For this review, take the finished solid that the model builds, in its own axes (mm). Coordinates: 2 decimals unless noted, no trailing zeros. Loops run counter-clockwise (first coordinate to the right, second up) from the corner with the lowest first, then second, coordinate; pieces in that order, holes last. Notation, with made-up numbers: (18, 22) -> (55, 22) arc R22 cw to (55, 34) -> close; hole circle Ø9 at (27, 53). An arc over 180 degrees is marked (long way). Answer in a Markdown table with one row per item.
from build123d import *

# Parameters (mm, degrees)
SKETCH_1_W          = 53
SKETCH_1_H          = 40
EXTRUDE_1_DEPTH     = 3
SKETCH_2_R          = 1.55
CUT_EXTRUDE_1_DEPTH = 10
SKETCH_4_R          = 1.65
CUT_EXTRUDE_2_DEPTH = 10
SKETCH_5_R          = 1.05
CUT_EXTRUDE_3_DEPTH = 10
SKETCH_6_W          = 23
SKETCH_6_H          = 12.5
CUT_EXTRUDE_4_DEPTH = 10
SKETCH_7_W          = 24
SKETCH_7_H          = 14
CUT_EXTRUDE_5_DEPTH = 10
SKETCH_8_W          = 40
SKETCH_8_H          = 10
CUT_EXTRUDE_6_DEPTH = 10
SKETCH_9_R          = 1.55
CUT_EXTRUDE_7_DEPTH = 10
FILLET_1_R          = 2


with BuildPart() as part:
    # 草图1 → 凸台-拉伸1 (new body)
    with BuildSketch(Plane(origin=(0, 0, 0), x_dir=(1, 0, 0), z_dir=(0, 1, 0))):
        Rectangle(SKETCH_1_W, SKETCH_1_H)
    extrude(amount=EXTRUDE_1_DEPTH)

    # 草图2 → 切除-拉伸1 (cut)
    with BuildSketch(Plane(origin=(0, 0, 0), x_dir=(-1, 0, 0), z_dir=(0, -1, 0))):
        with Locations(Location((20.5, -15, 0), (0, 0, 90))):
            Circle(SKETCH_2_R)
        with Locations(Location((20.5, 5, 0), (0, 0, 90))):
            Circle(SKETCH_2_R)
    extrude(amount=-CUT_EXTRUDE_1_DEPTH, mode=Mode.SUBTRACT)

    # 草图4 → 切除-拉伸2 (cut)
    with BuildSketch(Plane(origin=(0, 3, 0), x_dir=(1, 0, 0), z_dir=(0, 1, 0))):
        with Locations(Location((-8.5, -17, 0), (0, 0, 270))):
            Circle(SKETCH_4_R)
        with Locations(Location((11.5, -17, 0), (0, 0, 270))):
            Circle(SKETCH_4_R)
        with Locations(Location((-0.5, 17, 0), (0, 0, 270))):
            Circle(SKETCH_4_R)
        with Locations(Location((19.5, 17, 0), (0, 0, 270))):
            Circle(SKETCH_4_R)
    extrude(amount=-CUT_EXTRUDE_2_DEPTH, mode=Mode.SUBTRACT)

    # 草图5 → 切除-拉伸3 (cut)
    with BuildSketch(Plane(origin=(0, 3, 0), x_dir=(1, 0, 0), z_dir=(0, 1, 0))):
        with Locations(Location((22.599975, -7.75, 0), (0, 0, 270))):
            Circle(SKETCH_5_R)
        with Locations(Location((-5.100025, -7.75, 0), (0, 0, 270))):
            Circle(SKETCH_5_R)
    extrude(amount=-CUT_EXTRUDE_3_DEPTH, mode=Mode.SUBTRACT)

    # 草图6 → 切除-拉伸4 (cut)
    with BuildSketch(Plane(origin=(0, 0, 0), x_dir=(-1, 0, 0), z_dir=(0, -1, 0))):
        with Locations((-8.749975, -7.75)):
            Rectangle(SKETCH_6_W, SKETCH_6_H)
    extrude(amount=-CUT_EXTRUDE_4_DEPTH, mode=Mode.SUBTRACT)

    # 草图7 → 切除-拉伸5 (cut)
    with BuildSketch(Plane(origin=(0, 0, 0), x_dir=(-1, 0, 0), z_dir=(0, -1, 0))):
        with Locations((-8.749975, -7.75)):
            Rectangle(SKETCH_7_W, SKETCH_7_H)
    extrude(amount=-CUT_EXTRUDE_5_DEPTH, mode=Mode.SUBTRACT)

    # 草图8 → 切除-拉伸6 (cut)
    with BuildSketch(Plane(origin=(0, 0, 0), x_dir=(-1, 0, 0), z_dir=(0, -1, 0))):
        with Locations((-6.5, 15)):
            Rectangle(SKETCH_8_W, SKETCH_8_H)
    extrude(amount=-CUT_EXTRUDE_6_DEPTH, mode=Mode.SUBTRACT)

    # 草图9 → 切除-拉伸7 (cut)
    with BuildSketch(Plane(origin=(0, 0, 0), x_dir=(-1, 0, 0), z_dir=(0, -1, 0))):
        with Locations(Location((-11.5, 7, 0), (0, 0, 90))):
            Circle(SKETCH_9_R)
        with Locations(Location((8.5, 7, 0), (0, 0, 90))):
            Circle(SKETCH_9_R)
    extrude(amount=-CUT_EXTRUDE_7_DEPTH, mode=Mode.SUBTRACT)

    # 圆角1
    fillet_1_edges = [part.edges().sort_by_distance(p)[0] for p in [
        (26.5, 1.5, -10),
        (-13.5, 1.5, -20),
        (-13.5, 1.5, -10),
        (26.5, 1.5, 20),
        (-26.5, 1.5, 20),
        (-26.5, 1.5, -20),
    ]]
    fillet(fillet_1_edges, radius=FILLET_1_R)


solid = part.part
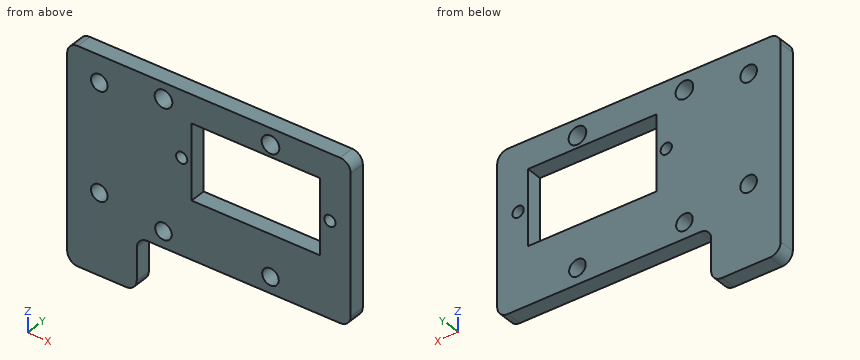
Item 1: Take a section at B-B, the plane x = 11.5. State the section outline as (y, z) points, and give its area (3 significant figures).
Worked answers:
| item | result |
|---|---|
| outline | (0, -10) -> (3, -10) -> (3, -8.55) -> (0, -8.55) -> close; (0, -5.45) -> (3, -5.45) -> (3, 0.75) -> (0, 0.75) -> close; (0, 14.75) -> (3, 14.75) -> (3, 15.35) -> (0, 15.35) -> close; (0, 18.65) -> (3, 18.65) -> (3, 20) -> (0, 20) -> close |
| area | 28.8 mm² |
Item 2: Take a section at A-A, the plane z = 10.5. State the section outline as (x, y) points, and give its area (3 significant figures).
Worked answers:
| item | result |
|---|---|
| outline | (-26.5, 0) -> (-3.25, 0) -> (-3.25, 3) -> (-26.5, 3) -> close; (20.75, 0) -> (26.5, 0) -> (26.5, 3) -> (20.75, 3) -> close |
| area | 87.0 mm² |
Item 3: For L1, parallel to X at y = 1.8, z = 7.75; L2, parallel to X at y = 1.75, z = 17; L3, parallel to X at y = 1.25, z = 15, list the stretches that pass through material, from the lowest coordinate up.
Worked answers:
| item | result |
|---|---|
| L1 | -26.5 to -6.15, -4.05 to -3.25, 20.75 to 21.55, 23.65 to 26.5 |
| L2 | -26.5 to -10.15, -6.85 to 9.85, 13.15 to 26.5 |
| L3 | -26.5 to -22.05, -18.95 to 26.5 |
Item 4: Take a section at C-C, the plane y = 2. Count the separate pieces of the cut face and the enclosed holes in it, and give its area (3 significant figures).
Worked answers:
| item | result |
|---|---|
| separate pieces | 1 |
| enclosed holes | 9 |
| area | 1,330 mm² |
Item 5: Insertion check: pin 1 (6 mm diameter, centred on x = -17, z = 14.5, fed in from -Y); pin 2 (0.9 mm diameter, centred on x = -1, y = 1.5, fed in from -Z); pin 3 (1.5 mm diameter, centred on y = 1.5, z = -15.5, fed in from +X). Each pin has a flat end and moves straight along its axis. Give the tip position at first contact, or say it passes through.
Worked answers:
| item | result |
|---|---|
| pin 1 | y = 0 |
| pin 2 | z = -10 |
| pin 3 | x = -13.5 |
Item 6: Take a section at D-D, the plane z = -15.5. State the section outline as (x, y) points.
Worked answers:
| item | result |
|---|---|
| outline | (-26.5, 0) -> (-13.5, 0) -> (-13.5, 3) -> (-26.5, 3) -> close |
